```python
from build123d import *

# Parameters (mm, degrees)
F0_R     = 12.7
F0_R_2   = 4.7625
F1_DEPTH = 15.875
F3_DEPTH = 9.525
F4_W     = 3.175
F4_H     = 3.175
F6_R     = 1.58749


# Not quite as in the source:
# - a fillet or chamfer is up to 0.001 mm smaller than in the source, because OpenCascade refuses the exact size


with BuildPart() as f1:
    # F0 (on Top) → F1 (new body)
    with BuildSketch(Plane.XY):
        Circle(F0_R)
        Circle(F0_R_2, mode=Mode.SUBTRACT)
        Circle(F0_R_2)
    extrude(amount=F1_DEPTH)

    # F0 (on Top) → F3 (join)
    with BuildSketch(Plane.XY):
        Circle(F0_R_2)
    extrude(amount=-F3_DEPTH)

    # F4 (on Right) → F5 (revolve, cut)
    with BuildSketch(Plane.YZ):
        with Locations((11.1125, 4.7625)):
            Rectangle(F4_W, F4_H)
        with Locations((11.1125, 11.1125)):
            Rectangle(F4_W, F4_H)
    revolve(axis=Axis((0, 0, -0.284396112), (0, 0, 1)), mode=Mode.SUBTRACT)

    # F6 (radius 1.5875 in the source; OpenCascade refuses exactly that, so slightly less here)
    f6_edges = [f1.edges().sort_by_distance(p)[0] for p in [
        (0, -9.525, 3.175),
        (0, -9.525, 6.35),
        (0, -9.525, 9.525),
        (0, -9.525, 12.7),
    ]]
    fillet(f6_edges, radius=F6_R)


solid = f1.part
```
CAD build for the part. Positions are in the model's coordinates, mm. A direction names the side the tool comes from. Coordinates: 2 decimals unless noted, no trailing zeros. Write each loop counter-clockwise with the first axis right and the second up, starting at its lowest first coordinate (ties: lowest second). Pieces come first, ordered by that corner, then holes.
(1) Flat gauge pins, fed straight in: pin 1 (6 mm diameter, centred on x = 2.5, z = 1, fed in from -Y); pin 2 (1.5 mm diameter, centred on x = -8, y = 4, fed in from -Z); pin 3 (5 mm diameter, centred on x = 5.5, z = -1.5, fed in from -Y); pin 4 (1 mm diameter, centred on y = 5.5, z = 3.5, fed in from -X). Where does each tip first touch, or does it go through?
(2) 3-axis set-ups, long thin cutter, end or side, ignore diameter. For faces 1 (the face through (11.23, -0.88, 6.35)), 2 (the face through (-3.78, -2.9, -4.7)), 3 (the face through (0, 0, 15.875)): which of +Z, -Z, +X, -X, +Y, -Y reach the whole face in a straight line?
(3) Drill centre lines: probe 1 along Z at (x, y) = (4.5, 10.5) (3 decimals); probe 2 along Z at (x, y) = (-10.25, 0.5) (3 decimals); probe 3 along Y at (x, z) = (0, 12.75). Where is each one in solid material? Low to high.
(4) Cut at C-C, the plane y = 10.5. Count the separate pieces of the cut face and the enclosed holes in it, and give its area (3 significant figures).
(5) Cut at D-D, the plane z = -5.5. List the corners of the cut face in (x, y) (1 decimal), and give its area (3 significant figures).
Geometry says:
1. pin 1: stops at y = -12.7
1. pin 2: stops at z = 0
1. pin 3: stops at y = -12.21
1. pin 4: stops at x = -11.62
2. face 1: none
2. face 2: -Z
2. face 3: +Z, +X, -X, +Y, -Y
3. probe 1: z = 0 to 3.175, 6.35 to 9.525, 12.7 to 15.875
3. probe 2: z = 0 to 3.422, 6.103 to 9.772, 12.453 to 15.875
3. probe 3: y = -12.7 to 12.7
4. separate pieces: 3
4. enclosed holes: 0
4. area: 138 mm2
5. outline: circle Ø9.5 at (0, 0)
5. area: 71.3 mm2
